Build history of the part. All positions in model axes, mm. A direction names the side the tool comes from. Give positions to 0.01 mm unless a question says otherwise; leave off trailing zeros. Order: outer loops, then holes, each group sorted by start corner. A loop starts at its lowest first (then second) coordinate and runs counter-clockwise, first axis right, second up. Notation, with made-up numbers: (14, 39.5) - (68, 39.5) arc R30 cw to (68, 71.5) - close; hole circle Ø6 at (-28.75, 84). An arc over 180 degrees is marked (long way). One line per item, written item: value.
Autodesk Inventor part; units mm, degrees
ref_plane "Work Plane1" through (-22.683, 21.414, 0) normal (0.5, 0.8660254, 0) x (-0.8660254, 0.5, 0)
ref_plane "YZ Plane" through (0, 0, 0) normal (1, 0, 0) x (0, 1, 0)
ref_plane "XZ Plane" through (0, 0, 0) normal (0, 1, 0) x (-1, 0, 0)
sketch "Sketch1" plane through (0, 0, 0) normal (0, 0, 1) x (1, 0, 0)
  line L0 (-19.508, -285.2191) -> (-19.508, 19.5809)
  line L1 (-19.508, 19.5809) -> (-52.5036, 38.6309)
  line L2 (-52.5036, 38.6309) -> (-55.6786, 33.1316)
  line L3 (-19.508, 19.5809) -> (-25.858, 15.9147)
  line L4 (-55.6786, 33.1316) -> (-25.858, 15.9147)
  line L5 (-25.858, 15.9147) -> (-25.858, -285.2191)
  line L6 (-25.858, -285.2191) -> (-19.508, -285.2191)
  point P0 (0, 0)
  dimension "d0" = 120
  dimension "d1" = 304.8
  dimension "d2" = 38.1
  dimension "d4" = 6.35
extrude "Extrusion1" add sketch "Sketch1" against normal blind 304.8
fillet "Fillet1" radius 6.35 2 edges at (-19.508, 19.5809, -152.4) (-25.858, 15.9147, -152.4)
sketch "Sketch2" plane through (-52.5036, 38.6309, 0) normal (0.5, 0.8660254, 0) x (0.8660254, -0.5, 0)
  line L0 (0, 0) -> (0, 304.8)
  line L1 (34.4338, 0) -> (0, 0)
  point P0 (64.7849, 0)
  point P1 (15.24, 50.8)
  point P2 (15.24, 254)
  dimension "d8" = 50.8
  dimension "d10" = 254
  dimension "d11" = 15.24
  dimension "d12" = 15.24
hole "Hole1" at (-39.3054, 31.0109, -50.8) at (-39.3054, 31.0109, -254) direction (-0.5, -0.8660254, 0) diameter 6.858 depth 25.4 tip angle 118
sketch "Sketch3" plane through (-25.858, -285.2191, 0) normal (0, -1, 0) x (1, 0, 0)
  line L0 (0, -304.8) -> (6.35, -304.8)
  line L1 (6.35, 0) -> (6.35, -304.8)
  line L2 (0, 0) -> (6.35, 0)
  line L3 (0, 0) -> (0, -304.8)
  line L4 (6.35, 0) -> (52.6401, 0)
  line L5 (52.6401, 0) -> (52.6401, -304.8)
  line L6 (52.6401, -304.8) -> (6.35, -304.8)
  line L7 (6.35, -304.8) -> (6.35, 0)
  line L8 (6.35, -6.35) -> (46.2901, -6.35)
  line L9 (46.2901, -6.35) -> (46.2901, -298.45)
  line L10 (46.2901, -298.45) -> (6.35, -298.45)
  line L11 (6.35, -298.45) -> (6.35, -6.35)
  point P0 (25.858, 0)
  dimension "d20" = 6.35
  dimension "d21" = 6.35
  dimension "d22" = 6.35
ref_plane "Work Plane1" through (-22.683, 21.414, 0) normal (0.5, 0.8660254, 0) x (-0.8660254, 0.5, 0)
extrude "Extrusion2" add sketch "Sketch3" against normal blind 266.7 contours L1 L10 L9 L8 L4 L5 L6
thread "Thread1"
thread "Thread2"
properties part number "slideFeeder"
(1) Pull direction Z, two halves, no side cores. Call faces 4 (the face through (0, -154, -6.35)), 5 (the face through (-39.78, 27.57, -47.63)), 6 (the face through (-6, -157, 0)), 7 (the face through (-6, -157, -304.8)): +Z half, -Z half, draft (parallel to the pull), parting line (faces both ways), or undercut.
Completed:
face 4: undercut
face 5: undercut
face 6: +Z half
face 7: -Z half
(2) Drill centre lines: line 1 (X direction, y = -139.5, z = -268); line 2 (Z direction, x = 6.5, y = -70.5); line 3 (Y direction, x = 21.5, z = -201.5). Where is each one in solid material? Low to high.
Completed:
line 1: -25.86 to -19.51, 20.43 to 26.78
line 2: -304.8 to -298.45, -6.35 to 0
line 3: -285.22 to -18.52
(3) Slice it at A-A, the plane x = 8. Give the cut face in (y, z).
Completed:
outline: (-285.22, -304.8) - (-18.52, -304.8) - (-18.52, -298.45) - (-285.22, -298.45) - close; (-285.22, -6.35) - (-18.52, -6.35) - (-18.52, 0) - (-285.22, 0) - close
(4) Slice it at B-B, the plane z = -110. Give the cut face in (x, y).
Completed:
outline: (-55.68, 33.13) - (-29.03, 17.75) arc R6.35 cw to (-25.86, 12.25) - (-25.86, -285.22) - (-19.51, -285.22) - (-19.51, 15.91) arc R6.35 ccw to (-22.68, 21.41) - (-52.5, 38.63) - close; (20.43, -285.22) - (26.78, -285.22) - (26.78, -18.52) - (20.43, -18.52) - close
(5) Pin check, flat tips, straight feed: P1, Ø1, axis at y = -250, z = -171.5, coming from the -X side; P2, Ø6, axis at x = -17, y = 3, coming from the -Z side; P3, Ø2, axis at x = -27, z = -35, coming from the +Y side. Stop position of each tip, or through.
Completed:
P1: x = -25.86
P2: z = -304.8
P3: y = 24.48
(6) Slice it at C-C, the plane y = -102.5. Give the cut face in (x, z).
Completed:
outline: (-25.86, -304.8) - (26.78, -304.8) - (26.78, 0) - (-25.86, 0) - close; hole (-19.51, -298.45) - (20.43, -298.45) - (20.43, -6.35) - (-19.51, -6.35) - close
(7) 3-axis set-ups, long thin cutter, end or side, ignore diameter. For faces 1 (the face through (1, -154, -298.45)), 2 (the face through (-25.858, -134, -150)), 3 (the face through (22, -18.519, -129)): which of +Z, -Z, +X, -X, +Y, -Y reach the whole face in a straight line?
Completed:
face 1: +Y, -Y
face 2: +Z, -Z, -X, -Y
face 3: +Z, -Z, +X, +Y
